from build123d import *

# Parameters (mm, degrees)
PAD001_DEPTH = 4
SKETCH_W     = 44
SKETCH_H     = 10
SKETCH_R     = 2
SKETCH_R_2   = 0.5
PAD_DEPTH    = 5
FILLET_R     = 4


with BuildPart() as body001:
    # Sketch001 → Pad001 (new body)
    with BuildSketch(Plane.XY):
        Polygon((0.897343, 1.560377), (1.338059, 1.486472), (1.457743, 1.055929), (1.827866, 0.81173), (1.760844, 0.373401), (2, 0), (1.760844, -0.373401), (1.827866, -0.81173), (1.457743, -1.055929), (1.341095, -1.483734), (0.903715, -1.556695), (0.623475, -1.900336), (0.194127, -1.789501), (-0.201465, -1.989827), (-0.548876, -1.714274), (-0.991727, -1.736801), (-1.1974, -1.343962), (-1.611279, -1.184813), (-1.63981, -0.742308), (-1.953475, -0.428878), (-1.799954, -0.012879), (-1.959412, 0.400881), (-1.650264, 0.718768), (-1.628067, 1.161635), (-1.216508, 1.32669), (-1.016478, 1.722432), (-0.569861, 1.707413), (-0.221793, 1.987664), (0.179488, 1.791029), (0.611809, 1.904124), align=None)
    extrude(amount=PAD001_DEPTH)


with BuildPart() as body001_1:
    # Body001 placement: moved
    add(body001.part.moved(Location((17, 0, -1))))


with BuildPart() as cut:
    # Sketch → Pad (new body)
    with BuildSketch(Plane.XY):
        Rectangle(SKETCH_W, SKETCH_H)
        with Locations((-17, 0)):
            Circle(SKETCH_R, mode=Mode.SUBTRACT)
        with Locations((17, 0)):
            Circle(SKETCH_R_2, mode=Mode.SUBTRACT)
    extrude(amount=PAD_DEPTH)

    # Fillet
    fillet_edges = [cut.edges().sort_by_distance(p)[0] for p in [
        (-22, 5, 2.5),
        (-22, -5, 2.5),
        (22, -5, 2.5),
        (22, 5, 2.5),
    ]]
    fillet(fillet_edges, radius=FILLET_R)

    # Cut: cut Body001
    add(body001_1.part, mode=Mode.SUBTRACT)


solid = cut.part
Here's how the part is built. I have some questions about the finished solid (model axes, mm). A direction names the side the tool comes from. Coordinates: 2 decimals unless noted, no trailing zeros. Loops run counter-clockwise (first coordinate to the right, second up) from the corner with the lowest first, then second, coordinate; pieces in that order, holes last. Notation, with made-up numbers: (-27.5, 47.5) -> (-11.5, 47.5) arc R19 ccw to (-11.5, 60.5) -> close; hole circle Ø9 at (66.25, 84). An arc over 180 degrees is marked (long way). Use one line per item in the form item = value. Start each with the question number.
(1) If we section it at A-A (x = -17): Please give me the cut outline in (y, z), then the cut area to 3 significant figures.
(2) On a 3-axis mill with a long thin cutter (end or side, diameter ignored), from which of +Z, -Z, +X, -X, +Y, -Y can I reach the whole of each face in a straight line? I mean faces 1 (the face through (17.5, 0.5, 3)), 2 (the face through (0, -5, 2)). Say none if no direction works.
(3) If we section it at B-B (z = 3.65): Please give me the cut outline in (x, y).
(4) If we section it at D-D (z = 1): Give the number of separate pieces and of enclosed holes in the cut face, then the cut area to 3 significant figures.
(5) We'd pull the mould along Y, two halves only. Please class faces 3 (the face through (-18.6, -1.2, 2.5)), 4 (the face through (-20.859, -3.797, 2.535)), 5 (the face through (0, 0, 0)): pulls with the +Y half, pulls with the -Y half, needs draft (parallel to the pull), parting line crosses it, or undercut.
(6) Please list where these lines run through material, in increasing order: line 1 along Y through (x, z) = (17, 3.4); line 2 along X through (y, z) = (-0.5, 2.45); line 3 along Y through (x, z) = (-17, 1.65).
(7) Will this pin go through, and if not, where does the flat tip stop? pin 1 (1.2 mm diameter, centred on x = 18, y = 0, fed in from -Z).
(8) If we section it at C-C (y = -3): Please give me the cut outline in (x, z), then the cut area to 3 significant figures.
Verdict:
q1.outline = (-5, 0) -> (-2, 0) -> (-2, 5) -> (-5, 5) -> close; (2, 0) -> (5, 0) -> (5, 5) -> (2, 5) -> close
q1.area = 30.0 mm²
q2.face_1 = -Z
q2.face_2 = +Z, -Z, +X, -X, -Y
q3.outline = (-22, -1) arc R4 ccw to (-18, -5) -> (18, -5) arc R4 ccw to (22, -1) -> (22, 1) arc R4 ccw to (18, 5) -> (-18, 5) arc R4 ccw to (-22, 1) -> close; hole circle Ø4 at (-17, 0); hole circle Ø1 at (17, 0)
q4.separate_pieces = 1
q4.enclosed_holes = 2
q4.area = 402 mm²
q5.face_3 = undercut
q5.face_4 = pulls with the -Y half
q5.face_5 = needs draft
q6.line_1 = -5 to -0.5, 0.5 to 5
q6.line_2 = -22 to -18.94, -15.06 to 15.12, 18.78 to 22
q6.line_3 = -5 to -2, 2 to 5
q7.pin_1 = 3
q8.outline = (-21.46, 0) -> (21.46, 0) -> (21.46, 5) -> (-21.46, 5) -> close
q8.area = 215 mm²
